Work out the finished part from the listing and answer in its coordinate system (mm). Face numbers are marked on the shaded views. A direction names the side the tool comes from. Give positions to 0.01 mm unless a question says otherwise; leave off trailing zeros. Loops run counter-clockwise (first coordinate to the right, second up) from the corner with the lowest first, then second, coordinate; pieces in that order, holes last. Notation, with made-up numbers: (-12, 37) - (46, 37) arc R30 cw to (46, 61) - close; hole circle Ø8 at (22, -29). An arc over 180 degrees is marked (long way). One line per question, with ' | ' between items. Start each with the question number.
1. Which of the six approach directions +Z, -Z, +X, -X, +Y, -Y give full straight-line access (tool end or side, diameter ignored) to the marked faces 1, 2 and 3?
2. Section A-A (x = -51) is taken. Determine the outline of the cut face in (y, z), plus the area to 3 significant figures.
3. Find the intervals of material crossed by line 1 (X direction, y = 34, z = 58); line 2 (Y direction, x = -17, z = 63); line 3 (Y direction, x = -18, z = 0) (3 decimals), in increasing order.
4. For a pull along Z with two mould halves and no side action, classify the marked faces 4, 5 and 6 as released by +Z, released by -Z, zero draft, split by the parting line, or undercut.
5. Each of these flat-tipped pins is pushed along its axis until it touches: pin 1 (25 mm diameter, centred on x = -32.385, y = 34.66, fed in from +Z); pin 2 (25 mm diameter, centred on y = -0.01, z = 63.5, fed in from +X); pin 3 (19 mm diameter, centred on x = -32.385, y = 34.66, fed in from +Z); pin 4 (1 mm diameter, centred on x = -12, y = 92.5, fed in from +Z). Where does it stop, or does it pass through?
6. Section B-B (z = 63.5) is taken. Give the number of separate pieces and of enclosed holes in the cut face, plus the area to 3 significant figures.
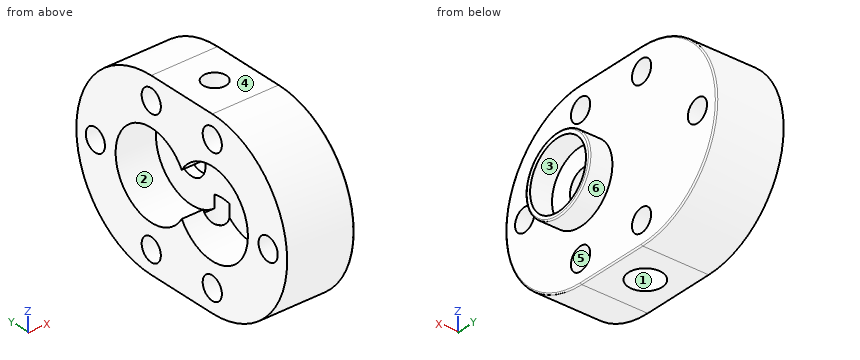
from build123d import *

# Parameters (mm, degrees)
BOSS_EXTRUDE1_DEPTH              = 63.5
SKETCH2_R                        = 10.9
CUT_EXTRUDE1_DEPTH               = 188.402765188
CUT_EXTRUDE2_DEPTH               = 38.1
SKETCH5_R                        = 36.195
BOSS_EXTRUDE2_DEPTH              = 21.59
F_97_2_5_DIAMETER_HOLE2_D        = 63.5
F_97_2_5_DIAMETER_HOLE2_DEPTH    = 20.69261314
F_97_2_5_DIAMETER_HOLE2_TIP      = 8.50738686
SKETCH11_R                       = 15.875
CUT_EXTRUDE3_DEPTH               = 183.470837396
F_97_1_25_DIAMETER_HOLE4_D       = 31.75
F_97_1_25_DIAMETER_HOLE4_DEPTH   = 9.24630657
F_97_1_25_DIAMETER_HOLE4_TIP     = 4.25369343
FILLET1_R                        = 1.27
F_1_16_1_25_DIAMETER_HOLE1_D     = 31.75
F_1_16_1_25_DIAMETER_HOLE1_DEPTH = 38.94630657
F_1_16_1_25_DIAMETER_HOLE1_TIP   = 4.25369343


with BuildPart() as part:
    # Sketch1 → Boss-Extrude1 (new body)
    with BuildSketch(Plane(origin=(0, 0, 0), x_dir=(0, 0, -1), z_dir=(1, 0, 0))):
        with BuildLine():
            Line((-85.1, 69.32), (-85.1, 0))
            ThreePointArc((-85.1, 0), (0, -85.1), (85.1, 0))
            Line((85.1, 0), (85.1, 69.32))
            ThreePointArc((85.1, 69.32), (0, 154.42), (-85.1, 69.32))
        make_face()
    extrude(amount=-BOSS_EXTRUDE1_DEPTH)

    # Sketch2 → Cut-Extrude1 (cut, through all)
    with BuildSketch(Plane(origin=(0, 0, 0), x_dir=(0, 0, -1), z_dir=(1, 0, 0))):
        with Locations((0, 132.83)):
            Circle(SKETCH2_R)
        with Locations((63.5, 69.33)):
            Circle(SKETCH2_R)
        with Locations(Location((-63.5, 69.33, 0), (0, 0, 180))):
            Circle(SKETCH2_R)
        with Locations(Location((63.5, -0.01, 0), (0, 0, 180))):
            Circle(SKETCH2_R)
        with Locations((-63.5, -0.01)):
            Circle(SKETCH2_R)
        with Locations(Location((0, -63.51, 0), (0, 0, 180))):
            Circle(SKETCH2_R)
    extrude(amount=-CUT_EXTRUDE1_DEPTH, mode=Mode.SUBTRACT)

    # Sketch3 → Cut-Extrude2 (cut)
    with BuildSketch(Plane.ZY.offset(63.5)):
        with BuildLine():
            ThreePointArc((-20.932552615, 34.671), (0, -40.5), (20.932552615, 34.671))
            ThreePointArc((20.932552615, 34.671), (0, 109.842), (-20.932552615, 34.671))
        make_face()
    extrude(amount=-CUT_EXTRUDE2_DEPTH, mode=Mode.SUBTRACT)

    # Sketch5 → Boss-Extrude2 (add)
    with BuildSketch(Plane(origin=(0, 0, 0), x_dir=(0, 0, -1), z_dir=(1, 0, 0))):
        Circle(SKETCH5_R)
    extrude(amount=BOSS_EXTRUDE2_DEPTH)

    # #97 (2.5) Diameter Hole2
    with Locations(Plane(origin=(21.59, 0.381274274, -0.515455507), x_dir=(0, 0, 1), z_dir=(1, 0, 0))):
        with Locations((0, 0)):
            Hole(F_97_2_5_DIAMETER_HOLE2_D / 2, depth=F_97_2_5_DIAMETER_HOLE2_DEPTH)
            with Locations((0, 0, -(F_97_2_5_DIAMETER_HOLE2_DEPTH + F_97_2_5_DIAMETER_HOLE2_TIP / 2))):  # 150° drill point
                Cone(0, F_97_2_5_DIAMETER_HOLE2_D / 2, F_97_2_5_DIAMETER_HOLE2_TIP, mode=Mode.SUBTRACT)

    # Sketch11 → Cut-Extrude3 (cut, through all)
    with BuildSketch(Plane.ZY.offset(25.4)):
        Circle(SKETCH11_R)
    extrude(amount=-CUT_EXTRUDE3_DEPTH, mode=Mode.SUBTRACT)

    # #97 (1.25) Diameter Hole4
    with Locations(Plane(origin=(-25.4, 69.342, 0), x_dir=(0, 0, -1), z_dir=(-1, 0, 0))):
        with Locations((0, 0)):
            Hole(F_97_1_25_DIAMETER_HOLE4_D / 2, depth=F_97_1_25_DIAMETER_HOLE4_DEPTH)
            with Locations((0, 0, -(F_97_1_25_DIAMETER_HOLE4_DEPTH + F_97_1_25_DIAMETER_HOLE4_TIP / 2))):  # 150° drill point
                Cone(0, F_97_1_25_DIAMETER_HOLE4_D / 2, F_97_1_25_DIAMETER_HOLE4_TIP, mode=Mode.SUBTRACT)

    # Fillet1
    fillet1_edges = [part.edges().sort_by_distance(p)[0] for p in [
        (0, 34.66, -85.1),
        (0, -85.1, 0),
        (0, 34.66, 85.1),
        (0, 154.42, 0),
        (21.59, 0, 36.195),
    ]]
    fillet(fillet1_edges, radius=FILLET1_R)

    # Sketch18 → 1/16 (0.86) Diameter Hole1 (revolve, cut)
    with BuildSketch(Plane(origin=(-32.385, 34.66, -85.1), x_dir=(0, 1, 0), z_dir=(1, 0, 0))):
        Polygon((0, 0), (0, 69), (10.922, 66.07345892), (10.922, 0), align=None)
    f_1_16_0_86_diameter_hole1 = revolve(axis=Axis((-32.385, 34.66, -91.45), (0, 0, 1)), mode=Mode.SUBTRACT)

    # Mirror1: 1/16 (0.86) Diameter Hole1 across plane
    add(f_1_16_0_86_diameter_hole1.mirror(Plane(origin=(0, 0, 0), x_dir=(1, 0, 0), z_dir=(0, 0, -1))), mode=Mode.SUBTRACT)

    # 1/16 (1.25) Diameter Hole1
    with Locations(Plane(origin=(-32.385, 34.66, -85.1), x_dir=(-1, 0, 0), z_dir=(0, 0, -1))):
        with Locations((0, 0)):
            Hole(F_1_16_1_25_DIAMETER_HOLE1_D / 2, depth=F_1_16_1_25_DIAMETER_HOLE1_DEPTH)
            with Locations((0, 0, -(F_1_16_1_25_DIAMETER_HOLE1_DEPTH + F_1_16_1_25_DIAMETER_HOLE1_TIP / 2))):  # 150° drill point
                Cone(0, F_1_16_1_25_DIAMETER_HOLE1_D / 2, F_1_16_1_25_DIAMETER_HOLE1_TIP, mode=Mode.SUBTRACT)


solid = part.part
Conclusion:
1) face 1: -Z | face 2: -X | face 3: +X
2) outline: (0, -85.1) - (69.32, -85.1) arc R85.1 ccw to (69.32, 85.1) - (0, 85.1) arc R85.1 ccw to start; hole circle Ø21.8 at (-63.51, 0); hole circle Ø21.8 at (-0.01, -63.5); hole circle Ø21.8 at (-0.01, 63.5); hole (34.67, -20.93) arc R40.5 ccw (long way) to (34.67, 20.93) arc R40.5 ccw (long way) to start; hole circle Ø21.8 at (69.33, -63.5); hole circle Ø21.8 at (69.33, 63.5); hole circle Ø21.8 at (132.83, 0) | area: 22,300 mm²
3) line 1: -63.5 to -43.29, -21.48 to 0 | line 2: -57.21 to -10.9, 10.88 to 58.44, 80.22 to 126.53 | line 3: -85.1 to -74.41, -52.61 to -15.875, 15.875 to 53.467, 85.217 to 121.93, 143.73 to 154.42
4) face 4: released by +Z | face 5: undercut | face 6: split by the parting line
5) pin 1: z = 85.1 | pin 2: x = 0 | pin 3: z = 18.65 | pin 4: z = 82.02
6) separate pieces: 3 | enclosed holes: 1 | area: 8,450 mm²
